from build123d import *

# Parameters (mm, degrees)
SKETCH1_R           = 7.5
BOSS_EXTRUDE1_DEPTH = 8
SKETCH2_R           = 4
SKETCH2_R_2         = 7.5
BOSS_EXTRUDE2_DEPTH = 2
SKETCH2_3_R         = 4
BOSS_EXTRUDE3_DEPTH = 17
SKETCH3_R           = 5
BOSS_EXTRUDE4_DEPTH = 13


with BuildPart() as part:
    # Sketch1 → Boss-Extrude1 (new body)
    with BuildSketch(Plane(origin=(0, 0, 0), x_dir=(1, 0, 0), z_dir=(0, 1, 0))):
        Circle(SKETCH1_R)
        Polygon((5.773502692, 0), (2.886751346, 5), (-2.886751346, 5), (-5.773502692, 0), (-2.886751346, -5), (2.886751346, -5), align=None, mode=Mode.SUBTRACT)
    extrude(amount=BOSS_EXTRUDE1_DEPTH)

    # Sketch2 → Boss-Extrude2 (add)
    with BuildSketch(Plane.XZ):
        Circle(SKETCH2_R)
        Circle(SKETCH2_R_2)
        Polygon((-2.886751346, 5), (2.886751346, 5), (5.773502692, 0), (2.886751346, -5), (-2.886751346, -5), (-5.773502692, 0), align=None, mode=Mode.SUBTRACT)
        Polygon((2.886751346, 5), (5.773502692, 0), (2.886751346, -5), (-2.886751346, -5), (-5.773502692, 0), (-2.886751346, 5), align=None)
        Circle(SKETCH2_R, mode=Mode.SUBTRACT)
        Circle(SKETCH2_R_2)
    extrude(amount=BOSS_EXTRUDE2_DEPTH)

    # Sketch2_3 → Boss-Extrude3 (add)
    with BuildSketch(Plane.XZ):
        Circle(SKETCH2_3_R)
    extrude(amount=BOSS_EXTRUDE3_DEPTH)

    # Sketch3 → Boss-Extrude4 (add)
    with BuildSketch(Plane.XZ.offset(17)):
        Circle(SKETCH3_R)
    extrude(amount=BOSS_EXTRUDE4_DEPTH)


solid = part.part
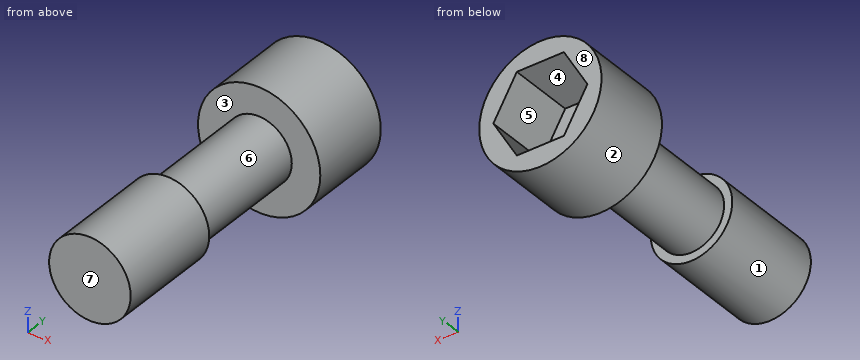
The listing builds one solid part. Answer for the finished solid, in the listing's coordinates (mm). Face numbers are marked on the shaded views. A direction names the side the tool comes from. Coordinates: 2 decimals unless noted, no trailing zeros. Write each loop counter-clockwise with the first axis right and the second up, starting at its lowest first coordinate (ties: lowest second). Pieces come first, ordered by that corner, then holes. Notation, with made-up numbers: M 86.25,-27.75 L 116.25,-27.75 A23 cw 116.25,-15.75 Z; hole C 68,20 d6. An arc over 180 degrees is marked long. Put each result on its own line as item: value. Start each with the question number.
1. A cutting plane is placed at D-D on z = -2.5. Write down the section's boundary in (x, y), then the cut area to 3 significant figures.
2. A cutting plane is placed at B-B on x = 0. Write down the section's boundary in (y, z), then the cut area to 3 significant figures.
3. A cutting plane is placed at C-C on y = -11. Write down the section's boundary in (x, z), then the cut area to 3 significant figures.
4. Consider line 1 (Y direction, x = -4.25, z = 2); line 2 (Y direction, x = 0.5, z = -6); line 3 (Y direction, x = -1.5, z = -0.25). Determine where each line is inside the solid, lowest interval first. Write a range as from..to.
5. Flat-ended cylindrical pins translate along their axes: P1, Ø1.5, axis at y = -6.5, z = 2.5, coming from the -X side; P2, Ø5, axis at x = -1, z = 0, coming from the +Y side; P3, Ø5, axis at x = -1, y = -17.5, coming from the -Z side. Find the tip coordinate at first contact, or state that the pin passes through.
6. Which of the six approach directions +Z, -Z, +X, -X, +Y, -Y give full straight-line access (tool end or side, diameter ignored) to the marked faces 1, 2, 3 and 4?
7. A cutting plane is placed at A-A on y = 0.5. Write down the section's boundary in (x, z), then the cut area to 3 significant figures.
8. For a pull along Y with two mould halves and no side action, classify the marked faces 5, 6, 7 and 8 as pulls with the +Y half, pulls with the -Y half, needs draft (parallel to the pull), parting line crosses it, or undercut.
Resolved:
1. outline: M -7.07,-2 L -3.12,-2 L -3.12,-17 L -4.33,-17 L -4.33,-30 L 4.33,-30 L 4.33,-17 L 3.12,-17 L 3.12,-2 L 7.07,-2 L 7.07,8 L 4.33,8 L 4.33,0 L -4.33,0 L -4.33,8 L -7.07,8 Z
1. area: 278 mm2
2. outline: M -30,-5 L -17,-5 L -17,-4 L -2,-4 L -2,-7.5 L 8,-7.5 L 8,-5 L 0,-5 L 0,5 L 8,5 L 8,7.5 L -2,7.5 L -2,4 L -17,4 L -17,5 L -30,5 Z
2. area: 320 mm2
3. outline: C 0,0 d8
3. area: 50.3 mm2
4. line 1: y = -30..-17, -2..0
4. line 2: y = -2..8
4. line 3: y = -30..0
5. P1: stops at x = -3.6
5. P2: stops at y = 0
5. P3: stops at z = -5
6. face 1: -Y
6. face 2: +Y, -Y
6. face 3: none
6. face 4: +Y
7. outline: C 0,0 d15; hole M -5.77,0 L -2.89,-5 L 2.89,-5 L 5.77,0 L 2.89,5 L -2.89,5 Z
7. area: 90.1 mm2
8. face 5: needs draft
8. face 6: undercut
8. face 7: pulls with the -Y half
8. face 8: pulls with the +Y half
